from build123d import *

# Parameters (mm, degrees)
SKETCH_1_R               = 5.5
EXTRUDE_1_DEPTH          = 14
SKETCH_2_R               = 3
CUT_EXTRUDE_1_DEPTH      = 17.015617378
CUT_EXTRUDE_2_DEPTH      = 17.015617378
CUT_EXTRUDE_2_DEPTH_BACK = 17.015617378
CUT_EXTRUDE_3_DEPTH      = 17.015617534
CUT_EXTRUDE_3_DEPTH_BACK = 17.015617534
FILLET_1_R               = 2.5
SKETCH_5_R               = 1.75
CUT_EXTRUDE_4_DEPTH      = 17.015617534
CUT_EXTRUDE_5_DEPTH      = 17.015617534
CUT_EXTRUDE_5_DEPTH_BACK = 17.015617534
SKETCH_6_R               = 1.4


with BuildPart() as part:
    # 草图1 → 凸台-拉伸1 (new body)
    with BuildSketch(Plane.XY):
        Circle(SKETCH_1_R)
    extrude(amount=EXTRUDE_1_DEPTH)

    # 草图2 → 切除-拉伸1 (cut, through all)
    with BuildSketch(Plane(origin=(0, 0, 0), x_dir=(-1, 0, 0), z_dir=(0, 0, -1))):
        Circle(SKETCH_2_R)
    extrude(amount=-CUT_EXTRUDE_1_DEPTH, mode=Mode.SUBTRACT)

    # 草图3 → 切除-拉伸2 (cut, two sides: drawn at the far end of the back side and taken through both)
    with BuildSketch(Plane(origin=(0, 0, 0), x_dir=(1, 0, 0), z_dir=(0, 1, 0)).offset(-CUT_EXTRUDE_2_DEPTH_BACK)):
        with BuildLine():
            Line((-3, -14), (3, -14))
            Line((3, -14), (3, -6.3))
            ThreePointArc((3, -6.3), (0, -4.3), (-3, -6.3))
            Line((-3, -6.3), (-3, -14))
        make_face()
    extrude(amount=CUT_EXTRUDE_2_DEPTH + CUT_EXTRUDE_2_DEPTH_BACK, mode=Mode.SUBTRACT)

    # 草图4 → 切除-拉伸3 (cut, two sides: drawn at the far end of the back side and taken through both)
    with BuildSketch(Plane(origin=(0, 0, 0), x_dir=(0, 0, -1), z_dir=(1, 0, 0)).offset(-CUT_EXTRUDE_3_DEPTH_BACK)):
        with BuildLine():
            Line((-14, 2.5), (-6.3, 2.5))
            ThreePointArc((-6.3, 2.5), (-4.003021048, 3.570262273), (-3.344955373, 6.017408205))
            Line((-3.344955373, 6.017408205), (-3.344955373, 8.923023013))
            Line((-3.344955373, 8.923023013), (-14, 8.923023013))
            Line((-14, 8.923023013), (-14, 2.5))
        make_face()
        with BuildLine():
            Line((-14, -2.5), (-6.3, -2.5))
            ThreePointArc((-6.3, -2.5), (-3.674156249, -4.049157281), (-3.760209141, -7.096703602))
            Line((-3.760209141, -7.096703602), (-6.538750291, -8.043650362))
            Line((-6.538750291, -8.043650362), (-14, -8.043650362))
            Line((-14, -8.043650362), (-14, -2.5))
        make_face()
    extrude(amount=CUT_EXTRUDE_3_DEPTH + CUT_EXTRUDE_3_DEPTH_BACK, mode=Mode.SUBTRACT)

    # 圆角1
    fillet_1_edges = [part.edges().sort_by_distance(p)[0] for p in [
        (-3.949489743, -2.5, 14),
        (-3.949489743, 2.5, 14),
        (3.949489743, 2.5, 14),
        (3.949489743, -2.5, 14),
    ]]
    fillet(fillet_1_edges, radius=FILLET_1_R - 0.0001)  # a hair under: the kernel refuses the full size

    # 草图5 → 切除-拉伸4 (cut, through all)
    with BuildSketch(Plane(origin=(0, 0, 0), x_dir=(0, 0, -1), z_dir=(1, 0, 0))):
        with Locations(Location((-2.8, 0, 0), (0, 0, 180))):
            Circle(SKETCH_5_R)
    extrude(amount=CUT_EXTRUDE_4_DEPTH, mode=Mode.SUBTRACT)

    # 草图6 → 切除-拉伸5 (cut, two sides: drawn at the far end of the back side and taken through both)
    with BuildSketch(Plane(origin=(0, 0, 0), x_dir=(0, 0, -1), z_dir=(1, 0, 0)).offset(-CUT_EXTRUDE_5_DEPTH_BACK)):
        with Locations((-11.8, 0)):
            Circle(SKETCH_6_R)
    extrude(amount=CUT_EXTRUDE_5_DEPTH + CUT_EXTRUDE_5_DEPTH_BACK, mode=Mode.SUBTRACT)


solid = part.part
CAD build for the part. Positions are in the model's coordinates, mm. A direction names the side the tool comes from. Round coordinates to 2 decimals unless told otherwise and drop trailing zeros. Write each loop counter-clockwise with the first axis right and the second up, starting at its lowest first coordinate (ties: lowest second). Pieces come first, ordered by that corner, then holes. Notation, with made-up numbers: M 35.25,87.25 L 60.25,87.25 A26 ccw 60.25,124.25 Z; hole C -14.5,34 d1. An arc over 180 degrees is marked long. Use a Markdown table: item, result. Add a question column.
1. Slice it at C-C on y = -2. Give the cut face in (x, z).
2. Flat gauge pins, fed straight in: P1, Ø5, axis at x = 1, y = 2.5, coming from the +Z side; P2, Ø2, axis at x = 3.5, z = 10, coming from the -Y side; P3, Ø0.9, axis at x = -4, z = 9, coming from the +Y side; P4, Ø2.5, axis at y = 0, z = 11.8, coming from the +X side. Where does each tip first touch, or does it go through?
3. Slice it at D-D on z = 11.8. Give the cut face in (x, y), then the cut area to 3 significant figures.
4. Slice it at B-B on x = 3.5. Give the number of separate pieces and of enclosed holes in the cut face, then the cut area to 3 significant figures.
5. Drill centre lines: probe 1 along Z at (x, y) = (-4.05, 0); probe 2 along X at (y, z) = (0, 2); probe 3 along Y at (x, z) = (-4.5, 13). Where is each one in solid material? Low to high.
6. Pull direction Y, two halves, no side cores. Call faces 5 (the face through (-4, 2.5, 9)), 6 (the face through (-4, -2.5, 9)), 7 (the face through (-4.27, 0.06, 13.2)): released by +Y, released by -Y, zero draft, split by the parting line, or undercut.
7. Slice it at A-A on z = 7. Give the cut face in (x, y).
8. 3-axis set-ups, long thin cutter, end or side, ignore diameter. For faces 1 (the face through (4, 2.5, 9)), 2 (the face through (3, 0, 9)), 3 (the face through (3.95, 1.71, 2.42)), 4 (the face through (4, -2.5, 9)): which of +Z, -Z, +X, -X, +Y, -Y reach the whole face in a straight line?
Reply:
| question | item | result |
|---|---|---|
| 1 | outline | M -5.12,0 L -2.24,0 L -2.24,5.19 A3.25 cw -3,6.3 L -3,13 L -5.12,13 Z; M 2.24,0 L 5.12,0 L 5.12,13 L 3,13 L 3,6.3 A3.25 cw 2.24,5.19 Z |
| 2 | P1 | stops at z = 13.79 |
| 2 | P2 | stops at y = -2.5 |
| 2 | P3 | stops at y = 2.5 |
| 2 | P4 | passes through |
| 3 | outline | M -5.32,-1.4 A5.5 ccw -4.91,-2.48 L -3,-2.48 L -3,-1.4 Z; M -5.32,1.4 L -3,1.4 L -3,2.48 L -4.91,2.48 A5.5 ccw Z; M 3,-2.48 L 4.91,-2.48 A5.5 ccw 5.32,-1.4 L 3,-1.4 Z; M 3,1.4 L 5.32,1.4 A5.5 ccw 4.91,2.48 L 3,2.48 Z |
| 3 | area | 9.24 mm^2 |
| 4 | separate pieces | 1 |
| 4 | enclosed holes | 2 |
| 4 | area | 66.7 mm^2 |
| 5 | probe 1 | z = 0 to 10.4, 13.2 to 14 |
| 5 | probe 2 | x = -5.5 to -3 |
| 5 | probe 3 | y = -2 to -0.72, 0.72 to 2 |
| 6 | face 5 | released by +Y |
| 6 | face 6 | released by -Y |
| 6 | face 7 | undercut |
| 7 | outline | M -4.9,-2.5 L -3,-2.5 L -3,2.5 L -4.9,2.5 A5.5 ccw Z; M 3,-2.5 L 4.9,-2.5 A5.5 ccw 4.9,2.5 L 3,2.5 Z |
| 8 | face 1 | +Z, +X, -X, +Y |
| 8 | face 2 | +Z, +Y, -Y |
| 8 | face 3 | +X |
| 8 | face 4 | +Z, +X, -X, -Y |
